CAD build for the part. Positions are in the model's coordinates, mm. A direction names the side the tool comes from. Coordinates: 2 decimals unless noted, no trailing zeros. Order: outer loops, then holes, each group sorted by start corner. A loop starts at its lowest first (then second) coordinate and runs counter-clockwise, first axis right, second up. Notation, with made-up numbers: (80, -16) - (123, -16) arc R28 ccw to (123, 13) - close; hole circle Ø7 at (30, 30.5). An arc over 180 degrees is marked (long way). Write each question's results on one line, items separated by ' | '. Start each with the question number.
Q1. Band-saw the part on A-A, the plane y = 121. Write the cut outline in (x, z).
Q2. Pin check, flat tips, straight feed: P1, Ø5.5, axis at y = 11.5, z = -9.5, coming from the -X side; P2, Ø2.5, axis at x = 6.01, z = 6.01, coming from the +Y side; P3, Ø4, axis at x = -4.5, y = 9, coming from the -Z side. Stop position of each tip, or through.
Q3. Wall check: probe 1 along Y at (x, z) = (-3, 2.5); probe 2 along Y at (x, z) = (-4, -5); probe 3 along Z at (x, y) = (-6.5, 134.5). Give the ranges that are in metal, low to high.
Q4. Which spindle directions (+Z, -Z, +X, -X, +Y, -Y) get a long thin tool onto all of the face, cutting with end or side? Do faces 1 (the flat face through (-5, 14, -5)), 2 (the flat face through (7, 11, -0.75)), 3 (the flat face through (-5, 15, 5)), 4 (the cylindrical face through (7.4, 145.01, 6.58)). Say none if no direction does.
Q5. Pull direction Y, two halves, no side cores. Call faces 5 (the flat face through (-7, 11, -0.75)), 6 (the cylindrical face through (-2.018, 144.986, -15.368)), 7 (the flat face through (0, 146, 0)): released by +Y, released by -Y, zero draft, split by the parting line, or undercut.
```python
from build123d import *

# Parameters (mm, degrees)
SKETCH1_R           = 13.5
BOSS_EXTRUDE1_DEPTH = 8
SKETCH3_R           = 12.5
BOSS_EXTRUDE3_DEPTH = 1
BOSS_EXTRUDE4_DEPTH = 135
SKETCH5_R           = 12.5
BOSS_EXTRUDE5_DEPTH = 1
SKETCH7_R           = 15.5
BOSS_EXTRUDE8_DEPTH = 2
SKETCH9_R           = 1.5
CUT_EXTRUDE1_DEPTH  = 2


with BuildPart() as part:
    # Sketch1 → Boss-Extrude1 (new body)
    with BuildSketch(Plane(origin=(0, 0, 0), x_dir=(1, 0, 0), z_dir=(0, 1, 0))):
        Circle(SKETCH1_R)
    extrude(amount=BOSS_EXTRUDE1_DEPTH)

    # Sketch3 → Boss-Extrude3 (add)
    with BuildSketch(Plane(origin=(0, 8, 0), x_dir=(1, 0, 0), z_dir=(0, 1, 0))):
        Circle(SKETCH3_R)
    extrude(amount=BOSS_EXTRUDE3_DEPTH)

    # Sketch4 → Boss-Extrude4 (add)
    with BuildSketch(Plane(origin=(0, 9, 0), x_dir=(1, 0, 0), z_dir=(0, 1, 0))):
        with BuildLine():
            Line((-0.75, -0.75), (-12.477479713, -0.75))
            ThreePointArc((-12.477479713, -0.75), (-12.5, 0), (-12.477479713, 0.75))
            Line((-12.477479713, 0.75), (-0.75, 0.75))
            Line((-0.75, 0.75), (-0.75, 12.477479713))
            ThreePointArc((-0.75, 12.477479713), (0, 12.5), (0.75, 12.477479713))
            Line((0.75, 12.477479713), (0.75, 0.75))
            Line((0.75, 0.75), (12.477479713, 0.75))
            ThreePointArc((12.477479713, 0.75), (12.5, 0), (12.477479713, -0.75))
            Line((12.477479713, -0.75), (0.75, -0.75))
            Line((0.75, -0.75), (0.75, -12.477479713))
            ThreePointArc((0.75, -12.477479713), (0, -12.5), (-0.75, -12.477479713))
            Line((-0.75, -12.477479713), (-0.75, -0.75))
        make_face()
    extrude(amount=BOSS_EXTRUDE4_DEPTH)

    # Sketch5 → Boss-Extrude5 (add)
    with BuildSketch(Plane(origin=(0, 14, 0), x_dir=(1, 0, 0), z_dir=(0, 1, 0))):
        Circle(SKETCH5_R)
    extrude(amount=BOSS_EXTRUDE5_DEPTH)

    # Sketch8 → Revolve1 (revolve)
    with BuildSketch(Plane.XY):
        Polygon((0, 0), (0, -7), (13.5, 0), align=None)
    revolve(axis=Axis((0, 0, 0), (0, -1, 0)))

    # Sketch7 → Boss-Extrude8 (add)
    with BuildSketch(Plane(origin=(0, 144, 0), x_dir=(1, 0, 0), z_dir=(0, 1, 0))):
        Circle(SKETCH7_R)
    extrude(amount=BOSS_EXTRUDE8_DEPTH)

    # Sketch9 → Cut-Extrude1 (cut)
    with BuildSketch(Plane(origin=(0, 146, 0), x_dir=(1, 0, 0), z_dir=(0, 1, 0))):
        with Locations((-6.01040764, 6.01040764)):
            Circle(SKETCH9_R)
        with Locations((6.01040764, 6.01040764)):
            Circle(SKETCH9_R)
        with Locations((6.01040764, -6.01040764)):
            Circle(SKETCH9_R)
        with Locations((-6.01040764, -6.01040764)):
            Circle(SKETCH9_R)
    extrude(amount=-CUT_EXTRUDE1_DEPTH, mode=Mode.SUBTRACT)


solid = part.part
```
Results below:
1) outline: (-12.48, -0.75) - (-0.75, -0.75) - (-0.75, -12.48) arc R12.5 ccw to (0.75, -12.48) - (0.75, -0.75) - (12.48, -0.75) arc R12.5 ccw to (12.48, 0.75) - (0.75, 0.75) - (0.75, 12.48) arc R12.5 ccw to (-0.75, 12.48) - (-0.75, 0.75) - (-12.48, 0.75) arc R12.5 ccw to start
2) P1: stops at x = -9.3 | P2: stops at y = 15 | P3: stops at z = -13.21
3) probe 1: y = -4.98 to 9, 14 to 15, 144 to 146 | probe 2: y = -3.68 to 9, 14 to 15, 144 to 146 | probe 3: z = -0.75 to 0.75
4) face 1: -Z, -X | face 2: -Z, +X | face 3: +Z, -X | face 4: +Y
5) face 5: undercut | face 6: zero draft | face 7: released by +Y
